Design review of the part built by this model. Coordinates are the model's own, in mm. A direction names the side the tool comes from. Round coordinates to 2 decimals unless told otherwise and drop trailing zeros. Order: outer loops, then holes, each group sorted by start corner. A loop starts at its lowest first (then second) coordinate and runs counter-clockwise, first axis right, second up.
Autodesk Inventor part; units mm, degrees
ref_plane "YZ Plane" through (0, 0, 0) normal (1, 0, 0) x (0, 1, 0)
ref_plane "XZ Plane" through (0, 0, 0) normal (0, 1, 0) x (-1, 0, 0)
ref_plane "XY Plane" through (0, 0, 0) normal (0, 0, 1) x (1, 0, 0)
sketch "Sketch1" plane through (0, 0, 0) normal (0, 1, 0) x (-1, 0, 0)
  line L0 (-102.1567, -250.3174) -> (-102.1567, 267.6805)
  line L1 (-102.1567, -246.3184) -> (-102.1567, 262.6816)
  line L2 (-102.1567, 262.6816) -> (14.8433, 262.6816)
  line L3 (102.8433, 80.6816) -> (14.8433, 168.6816)
  line L4 (14.8433, 262.6816) -> (14.8433, 168.6816)
  line L5 (14.8433, 168.6816) -> (102.8433, 80.6816)
  line L6 (102.8433, 80.6816) -> (102.8433, -65.3184)
  line L7 (102.8433, -65.3184) -> (14.8433, -153.3184)
  line L8 (14.8433, -153.3184) -> (14.8433, -246.3184)
  line L9 (14.8433, -246.3184) -> (-102.1567, -246.3184)
  point P0 (0, 0)
  point P1 (-37.1567, -11.3184)
  dimension "d0" = 509
  dimension "d1" = 117
  dimension "d2" = 117
  dimension "d3" = 93
  dimension "d4" = 94
  dimension "d6" = 88
  dimension "d7" = 88
  dimension "d8" = 88
  dimension "d9" = 88
extrude "Extrusion1" add sketch "Sketch1" along normal blind 10
sketch "Sketch2" plane through (0, 10, 0) normal (0, 1, 0) x (1, 0, 0)
  line L0 (-102.8433, 65.3184) -> (-102.8433, -80.6816)
  circle A0 centre (-102.8433, -7.6816) radius 9.3184
  circle A1 centre (-7.8433, -7.6816) radius 32.5
  circle A2 centre (-7.8433, -7.6816) radius 6.25
  line L1 (102.1567, -262.6816) -> (102.1567, 246.3184)
  line L2 (102.1567, 246.3184) -> (-14.8433, 246.3184)
  point P0 (0, 0)
  dimension "d14" = 95
  dimension "d16" = 254
  dimension "d17" = 110
  dimension "d18" = 65
  dimension "d19" = 12.5
extrude "Extrusion2" add sketch "Sketch2" along normal blind 39 contours A1
properties part number "XAxisCreplCaretki" material "Aluminum 6061"
1) Take a section at C-C on x = 4.5. Give the boundary of the cut face in (y, z).
Results:
outline: (0, -246.32) - (10, -246.32) - (10, -22.38) - (49, -22.38) - (49, 37.75) - (10, 37.75) - (10, 262.68) - (0, 262.68) - close
2) Clearance check with flat-ended pins moving along their axes: P1, Ø14.5, axis at x = -7.84, z = 7.68, coming from the -Y side; P2, Ø11, axis at y = 6, z = 194.5, coming from the -X side; P3, Ø1.5, axis at x = -61.5, z = 108.5, coming from the +Y side; P4, Ø1, axis at y = 28, z = 27, coming from the +X side. State where each tip first meets the part, or that it passes through.
Results:
P1: stops at y = 0
P2: stops at x = -14.84
P3: stops at y = 10
P4: stops at x = 18.65
3) To check wall thickness, follow line 1 along Y through (x, z) = (-67.5, -62.5); line 2 along Z through (x, y) = (-12, 44.5); line 3 along X through (y, z) = (8, -176.5). State the ranges of each line that lie inside material, in increasing order.
Results:
line 1: y = 0 to 10
line 2: z = -24.55 to 3.01, 12.35 to 39.91
line 3: x = -14.84 to 102.16
4) Take a section at D-D on y = 31. Give the boundary of the cut face in (x, z).
Results:
outline: circle Ø65 at (-7.84, 7.68); hole circle Ø12.5 at (-7.84, 7.68)
5) Take a section at B-B on z = -178. Give the boundary of the cut face in (x, y).
Results:
outline: (-14.84, 0) - (102.16, 0) - (102.16, 10) - (-14.84, 10) - close
6) For faces 1 (the face through (-14.843, 5, -199)), 2 (the face through (23.156, 29.227, 17.444)), 3 (the face through (-59.459, 4.93, 124.066)), list the 3-axis set-ups (+Z, -Z, +X, -X, +Y, -Y) from which the entire face can be reached by the end or side of a thin tool; tool diameter is ignored.
Results:
face 1: -Z, -X, +Y, -Y
face 2: +Y
face 3: +Z, -X, +Y, -Y
7) Take a section at A-A on y = 5. Give the boundary of the cut face in (x, z), plus the area to 3 significant figures.
Results:
outline: (-102.84, -65.32) - (-14.84, -153.32) - (-14.84, -246.32) - (102.16, -246.32) - (102.16, 262.68) - (-14.84, 262.68) - (-14.84, 168.68) - (-102.84, 80.68) - close
area: 80,100 mm2
8) The part is to be moulded in two halves that separate along X. For faces 4 (the face through (24, 0, 12)), 5 (the face through (-12.803, 29.227, 3.879)), 6 (the face through (-14.843, 5, 216)), say which applies: released by +X, released by -X, zero draft, split by the parting line, or undercut.
Results:
face 4: zero draft
face 5: undercut
face 6: released by -X
